from build123d import *

# Parameters (mm, degrees)
F0_W     = 70
F0_H     = 40
F1_DEPTH = 20
F2_W     = 60
F2_H     = 30
F3_DEPTH = 15
F4_W     = 59
F4_H     = 29
F5_DEPTH = 10


with BuildPart() as f1:
    # F0 (on Right) → F1 (new body)
    with BuildSketch(Plane.YZ):
        with Locations((35, 20)):
            Rectangle(F0_W, F0_H)
    extrude(amount=F1_DEPTH)

    # F2 (on face) → F3 (cut)
    with BuildSketch(Plane.YZ.offset(20)):
        with Locations((35, 20)):
            Rectangle(F2_W, F2_H)
    extrude(amount=-F3_DEPTH, mode=Mode.SUBTRACT)

    # F4 (on face) → F5 (join)
    with BuildSketch(Plane(origin=(0, 0, 0), x_dir=(0, -1, 0), z_dir=(-1, 0, 0))):
        with Locations((-35, 20)):
            Rectangle(F4_W, F4_H)
    extrude(amount=F5_DEPTH)


solid = f1.part
Build history of the part. All positions in model axes, mm. A direction names the side the tool comes from. Coordinates: 2 decimals unless noted, no trailing zeros. Write each loop counter-clockwise with the first axis right and the second up, starting at its lowest first coordinate (ties: lowest second). Pieces come first, ordered by that corner, then holes.
(1) Drill centre lines: line 1 (Z direction, x = 10, y = 60); line 2 (Y direction, x = 9.75, z = 10); line 3 (Z direction, x = -6.75, y = 45.5). Where is each one in solid material? Low to high.
(2) Cut at A-A on x = 13. List the corners of the cut face in (y, z), and give its area (3 significant figures).
(3) Cut at B-B on y = 9. List the corners of the cut face in (x, z), and give its area (3 significant figures).
(4) Cut at C-C on z = 23. List the corners of the cut face in (x, y), and give its area (3 significant figures).
(5) Pin check, flat tips, straight feed: pin 1 Ø3 at (x, z) = (-7, 16) entering from -Y; pin 2 Ø5 at (x, z) = (-6.5, 17) entering from +Y; pin 3 Ø8 at (x, y) = (-3, 34) entering from +Z; pin 4 Ø11 at (x, y) = (-6.5, 39) entering from +Z. Stop position of each tip, or through.
(6) 3-axis set-ups, long thin cutter, end or side, ignore diameter. For faces 5 (the flat face through (-5, 5.5, 20)), 6 (the flat face through (-5, 64.5, 20)), 7 (the flat face through (13, 5, 20)): which of +Z, -Z, +X, -X, +Y, -Y reach the whole face in a straight line?
(7) Cut at D-D on z = 3.5. List the corners of the cut face in (x, y), and give its area (3 significant figures).
(8) Mould opens along Y. For faces 1 (the flat face through (5, 35, 20)), 2 (the flat face through (10, 70, 20)), 3 (the flat face through (10, 35, 40)), 4 (the flat face through (10, 0, 20)) say: pulls with the +Y half, pulls with the -Y half, needs draft (parallel to the pull), parting line crosses it, or undercut.
Working result:
1. line 1: z = 0 to 5, 35 to 40
1. line 2: y = 0 to 5, 65 to 70
1. line 3: z = 5.5 to 34.5
2. outline: (0, 0) - (70, 0) - (70, 40) - (0, 40) - close; hole (5, 5) - (65, 5) - (65, 35) - (5, 35) - close
2. area: 1,000 mm2
3. outline: (-10, 5.5) - (0, 5.5) - (0, 0) - (20, 0) - (20, 5) - (5, 5) - (5, 35) - (20, 35) - (20, 40) - (0, 40) - (0, 34.5) - (-10, 34.5) - close
3. area: 640 mm2
4. outline: (-10, 5.5) - (0, 5.5) - (0, 0) - (20, 0) - (20, 5) - (5, 5) - (5, 65) - (20, 65) - (20, 70) - (0, 70) - (0, 64.5) - (-10, 64.5) - close
4. area: 1,090 mm2
5. pin 1: stops at y = 5.5
5. pin 2: stops at y = 64.5
5. pin 3: stops at z = 40
5. pin 4: stops at z = 34.5
6. face 5: +Z, -Z, -X, -Y
6. face 6: +Z, -Z, -X, +Y
6. face 7: +X
7. outline: (0, 0) - (20, 0) - (20, 70) - (0, 70) - close
7. area: 1,400 mm2
8. face 1: undercut
8. face 2: pulls with the +Y half
8. face 3: needs draft
8. face 4: pulls with the -Y half
